```python
from build123d import *

# Parameters (mm, degrees)
SKETCH1_R   = 9.525
SKETCH1_R_2 = 7.874


with BuildPart() as part:
    # Sweep1: sweep along a path in Sketch2
    with BuildLine(Plane.XY) as sweep1_path:
        Line((0, 0), (0, 12.7))
        ThreePointArc((0, 12.7), (6.932124101, 35.595250599), (25.4, 50.8))
        ThreePointArc((25.4, 50.8), (43.867875899, 66.004749401), (50.8, 88.9))
        Line((50.8, 88.9), (50.8, 101.6))
    # Sketch1 → Sweep1 (sweep)
    with BuildSketch(Plane(origin=(0, 0, 0), x_dir=(1, 0, 0), z_dir=(0, 1, 0))):
        Circle(SKETCH1_R)
        Circle(SKETCH1_R_2, mode=Mode.SUBTRACT)
    sweep(path=sweep1_path.line)


solid = part.part
```
The model under review builds one solid part; all positions refer to its coordinate system, in mm. A direction names the side the tool comes from. Give positions to 0.01 mm unless a question says otherwise; leave off trailing zeros. Write each loop counter-clockwise with the first axis right and the second up, starting at its lowest first coordinate (ties: lowest second). Pieces come first, ordered by that corner, then holes. Notation, with made-up numbers: M 58,-31 L 63,-31 A13 ccw 63,-7 Z; hole C 21,-36 d2. An arc over 180 degrees is marked long. Answer in a Markdown table with one row per item.
Item 1: For P1, Ø5, axis at x = 11, y = 44.5, coming from the +Z side; P2, Ø3, axis at x = 22, y = 57.5, coming from the -Z side; P3, Ø2, axis at x = 18, y = 49.5, coming from the -Z side; P4, Ø8, axis at x = 49, z = 5, coming from the -Y side, all flat-tipped, find the tip position at first contact; note any pin that passes through.
Check sheet entries:
| item | result |
|---|---|
| P1 | z = 9.52 |
| P2 | z = -7.4 |
| P3 | z = -9.44 |
| P4 | y = 53.75 |
Item 2: Add section B-B on y = 95. Give the boundary of the cut face in (x, z) (3 decimals), plus the area to 3 significant figures.
Check sheet entries:
| item | result |
|---|---|
| outline | C 50.8,0 d19.05; hole C 50.8,0 d15.748 |
| area | 90.2 mm2 |
Item 3: Add section A-A on z = 0. Give the boundary of the cut face in (x, y) (3 decimals), plus the area to 3 significant figures.
Check sheet entries:
| item | result |
|---|---|
| outline | M -9.525,0 L -7.874,0 L -7.874,12.7 A49.149 cw 22.372,58.068 A33.401 ccw 42.926,88.9 L 42.926,101.6 L 41.275,101.6 L 41.275,88.9 A31.75 cw 21.737,59.592 A50.8 ccw -9.525,12.7 Z; M 7.874,0 L 9.525,0 L 9.525,12.7 A31.75 cw 29.063,42.008 A50.8 ccw 60.325,88.9 L 60.325,101.6 L 58.674,101.6 L 58.674,88.9 A49.149 cw 28.428,43.532 A33.401 ccw 7.874,12.7 Z |
| area | 404 mm2 |
Item 4: For line 1 along Z through (x, y) = (50.8, 96.75) (3 decimals); line 2 along X through (y, z) = (97, 0) (3 decimals), list the stretches that pass through material, from the lowest coordinate up.
Check sheet entries:
| item | result |
|---|---|
| line 1 | -9.525 to -7.874, 7.874 to 9.525 |
| line 2 | 41.275 to 42.926, 58.674 to 60.325 |
Item 5: Tool access review of faces 1 (the face through (-1.707, 6.439, 7.687)), 2 (the face through (7, 0, -4)), 3 (the face through (59.6, 95.34, 3.65)): name each direction out of +Z, -Z, +X, -X, +Y, -Y from which nothing blocks a thin tool from reaching the whole face with its end or side.
Check sheet entries:
| item | result |
|---|---|
| face 1 | -Y |
| face 2 | +Z, -Z, +X, -X, -Y |
| face 3 | +Y |
Item 6: Draft analysis for pull direction X (two halves, no side actions). For faces 4 (the face through (58, 101.6, -4)), 5 (the face through (42.934, 95.339, -0.346)), 6 (the face through (-7.559, 6.439, 5.796)), state which applies: +X half, -X half, draft (parallel to the pull), parting line (faces both ways), or undercut.
Check sheet entries:
| item | result |
|---|---|
| face 4 | draft |
| face 5 | undercut |
| face 6 | parting line |
Item 7: Add section C-C on z = 6.75. Give the boundary of the cut face in (x, y) (3 decimals).
Check sheet entries:
| item | result |
|---|---|
| outline | M -6.72,0 L -4.054,0 L -4.054,12.7 A45.329 cw 23.841,54.542 A37.221 ccw 46.746,88.9 L 46.746,101.6 L 44.08,101.6 L 44.08,88.9 A34.555 cw 22.815,57.003 A47.995 ccw -6.72,12.7 Z; M 4.054,0 L 6.72,0 L 6.72,12.7 A34.555 cw 27.985,44.597 A47.995 ccw 57.52,88.9 L 57.52,101.6 L 54.854,101.6 L 54.854,88.9 A45.329 cw 26.959,47.058 A37.221 ccw 4.054,12.7 Z |
